CAD build for the part. Positions are in the model's coordinates, mm. A direction names the side the tool comes from. Round coordinates to 2 decimals unless told otherwise and drop trailing zeros. Loops run counter-clockwise (first coordinate to the right, second up) from the corner with the lowest first, then second, coordinate; pieces in that order, holes last. Notation, with made-up numbers: M -4,8.25 L 38,8.25 A21 cw 38,26.25 Z; hole C 38,-26.75 d3. An arc over 180 degrees is marked long. Use a Markdown table: item, result. Add a question column.
(1) Band-saw the part on D-D, the plane z = 32. Write the cut outline in (x, y).
(2) Band-saw the part on B-B, the plane y = -11. Write the cut outline in (x, z), and give its area (3 significant figures).
(3) Band-saw the part on A-A, the plane x = 0. Write the cut outline in (y, z), and give its area (3 significant figures).
(4) Wall check: L1, parallel to Y at x = -11, z = 28; L2, parallel to Y at x = 0, z = 31.25; L3, parallel to Y at x = -10.5, z = 10. Give the ranges that are in metal, low to high.
(5) Two-plate mould, pull along X, no slides. Class faces 3 (the face through (-1, 1, 0)), 4 (the face through (-8.67, -39.05, 17.26)), 5 (the face through (11.3, 15.23, 14.45)): released by +X, released by -X, zero draft, split by the parting line, or undercut.
(6) Flat gauge pins, fed straight in: P1, Ø10, axis at y = -20.5, z = 16, coming from the -X side; P2, Ø2, axis at x = -10.5, z = 9.5, coming from the -Y side; P3, Ø6, axis at x = -30, z = 30.5, coming from the -Y side. Where does each tip first touch, or does it go through?
(7) Which spindle directions (+Z, -Z, +X, -X, +Y, -Y) get a long thin tool onto all of the face, cutting with end or side? Do faces 1 (the face through (-15.89, -12.18, 31.8)), 2 (the face through (15.23, -11.3, 14.45)). Say none if no direction does.
from build123d import *

# Parameters (mm, degrees)
SKETCH1_R           = 40
BOSS_EXTRUDE1_DEPTH = 35
SKETCH2_R           = 20.02
CUT_EXTRUDE2_DEPTH  = 6.5
SKETCH3_R           = 5
CUT_EXTRUDE3_DEPTH  = 67.520673478
CIRPATTERN1_COUNT   = 4


with BuildPart() as part:
    # Sketch1 → Boss-Extrude1 (new body)
    with BuildSketch(Plane.XY):
        Circle(SKETCH1_R)
    extrude(amount=BOSS_EXTRUDE1_DEPTH)

    # Sketch2 → Cut-Extrude2 (cut)
    with BuildSketch(Plane.XY.offset(35)):
        Circle(SKETCH2_R)
    extrude(amount=-CUT_EXTRUDE2_DEPTH, mode=Mode.SUBTRACT)

    # Sketch3 → Cut-Extrude3 (cut, through all)
    with BuildSketch(Plane.XY.offset(35)):
        with Locations((-11.545851026, 7.917911598)):
            Circle(SKETCH3_R)
    cut_extrude3 = extrude(amount=-CUT_EXTRUDE3_DEPTH, mode=Mode.SUBTRACT)

    # CirPattern1: Cut-Extrude3 ×4 about axis
    cirpattern1_axis = Axis((0, 0, 0), (0, 0, 1))
    for i in range(1, CIRPATTERN1_COUNT):
        add(cut_extrude3.rotate(cirpattern1_axis, i * 360 / CIRPATTERN1_COUNT), mode=Mode.SUBTRACT)


solid = part.part
Return value:
| question | item | result |
|---|---|---|
| 1 | outline | C 0,0 d80; hole C 0,0 d40.04 |
| 2 | outline | M -38.46,0 L -12.89,0 L -12.89,28.5 L -16.73,28.5 L -16.73,35 L -38.46,35 Z; M -2.95,0 L 7.61,0 L 7.61,28.5 L -2.95,28.5 Z; M 15.48,0 L 38.46,0 L 38.46,35 L 16.73,35 L 16.73,28.5 L 15.48,28.5 Z |
| 2 | area | 1,970 mm^2 |
| 3 | outline | M -40,0 L 40,0 L 40,35 L 20.02,35 L 20.02,28.5 L -20.02,28.5 L -20.02,35 L -40,35 Z |
| 3 | area | 2,540 mm^2 |
| 4 | L1 | -38.46 to -15.48, -7.61 to 2.95, 12.89 to 38.46 |
| 4 | L2 | -40 to -20.02, 20.02 to 40 |
| 4 | L3 | -38.6 to -15.83, -7.26 to 3.03, 12.81 to 38.6 |
| 5 | face 3 | zero draft |
| 5 | face 4 | split by the parting line |
| 5 | face 5 | undercut |
| 6 | P1 | x = -36.87 |
| 6 | P2 | y = -38.86 |
| 6 | P3 | y = -29.51 |
| 7 | face 1 | +Z |
| 7 | face 2 | +Z, -Z |
